Design review of the part built by this model. Coordinates are the model's own, in mm. Face numbers are marked on the shaded views. A direction names the side the tool comes from. Give positions to 0.01 mm unless a question says otherwise; leave off trailing zeros. Loops run counter-clockwise (first coordinate to the right, second up) from the corner with the lowest first, then second, coordinate; pieces in that order, holes last.
from build123d import *

# Parameters (mm, degrees)
F0_W                 = 400
F0_H                 = 200
F1_DEPTH             = 3.6
F3_W                 = 400
F3_H                 = 200
F3_W_2               = 380
F3_H_2               = 180
F4_DEPTH             = 56.4
F7_D                 = 4.2
F7_DEPTH             = 12
F7_CBORE_D           = 8
F7_CBORE_DEPTH       = 4
F7_TIP               = 1.2618073
F7_ON_F5_D           = 4.2
F7_ON_F5_DEPTH       = 12
F7_ON_F5_CBORE_D     = 8
F7_ON_F5_CBORE_DEPTH = 4
F7_ON_F5_TIP         = 1.2618073


with BuildPart() as f1:
    # F0 (on Top) → F1 (new body)
    with BuildSketch(Plane.XY):
        Rectangle(F0_W, F0_H)
    extrude(amount=-F1_DEPTH)

    # F3 (on offset) → F4 (join, through all)
    with BuildSketch(Plane.XY.offset(-60)):
        Rectangle(F3_W, F3_H)
        Rectangle(F3_W_2, F3_H_2, mode=Mode.SUBTRACT)
    extrude(amount=F4_DEPTH)

    # F7
    with Locations(Plane(origin=(-200, 0, 0), x_dir=(0, -1, 0), z_dir=(-1, 0, 0))):
        with Locations((-75, -30), (75, -30)):
            CounterBoreHole(F7_D / 2, F7_CBORE_D / 2, F7_CBORE_DEPTH, depth=F7_DEPTH)
            with Locations((0, 0, -(F7_DEPTH + F7_TIP / 2))):  # 118° drill point
                Cone(0, F7_D / 2, F7_TIP, mode=Mode.SUBTRACT)

    # F7 on F5
    with Locations(Plane.YZ.offset(200)):
        with Locations((75, -30), (-75, -30)):
            CounterBoreHole(F7_ON_F5_D / 2, F7_ON_F5_CBORE_D / 2, F7_ON_F5_CBORE_DEPTH, depth=F7_ON_F5_DEPTH)
            with Locations((0, 0, -(F7_ON_F5_DEPTH + F7_ON_F5_TIP / 2))):  # 118° drill point
                Cone(0, F7_ON_F5_D / 2, F7_ON_F5_TIP, mode=Mode.SUBTRACT)


solid = f1.part
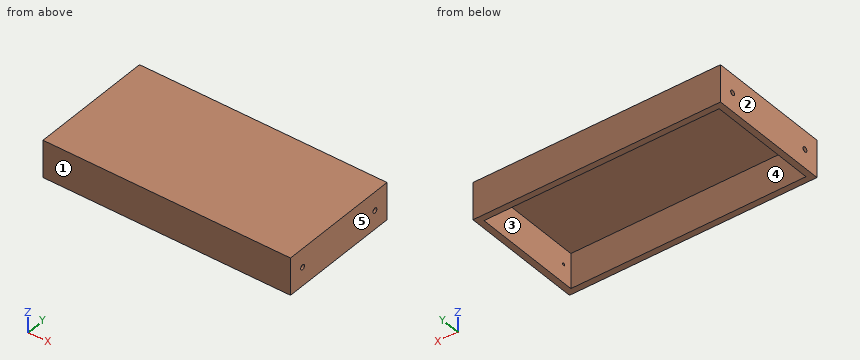
Q1. Take a section at A-A (y = -60.5). Give the boundary of the cut face in (x, z).
Results:
outline: (-200, -60) - (-190, -60) - (-190, -3.6) - (190, -3.6) - (190, -60) - (200, -60) - (200, 0) - (-200, 0) - close
Q2. Insertion check: pin 1 (4 mm diameter, centred on y = 75, z = -30, fed in from -X); pin 2 (2.5 mm diameter, centred on y = 74.5, z = -31, fed in from -X); pin 3 (6.5 mm diameter, centred on y = -75, z = -30, fed in from +X); pin 4 (8 mm diameter, centred on x = 145.5, y = 43, fed in from -Z). Each pin has a flat end and moves straight along its axis. Give the tip position at first contact, or say it passes through.
Results:
pin 1: passes through
pin 2: stops at x = -196
pin 3: stops at x = 196
pin 4: stops at z = -3.6
Q3. Wall thickness on line 1 (X direction, y = 14, z = -40); line 2 (Z direction, x = 192, y = 75); line 3 (Y direction, x = 65.5, z = -7.5): over which ranges is each line inside the solid? List them lowest first.
Results:
line 1: x = -200 to -190, 190 to 200
line 2: z = -60 to -32.1, -27.9 to 0
line 3: y = -100 to -90, 90 to 100
Q4. Draft analysis for pull direction Y (two halves, no side actions). For the marked faces 1, 2 and 3, state which applies: pulls with the +Y half, pulls with the -Y half, needs draft (parallel to the pull), parting line crosses it, or undercut.
Results:
face 1: pulls with the -Y half
face 2: needs draft
face 3: undercut
Q5. Tool access review of the marked faces 4 and 5: name each direction out of +Z, -Z, +X, -X, +Y, -Y from which nothing blocks a thin tool from reaching the whole face with its end or side.
Results:
face 4: -Z
face 5: +Z, -Z, +X, +Y, -Y
Q6. Take a section at C-C (x = -34). Give the boundary of the cut face in (y, z).
Results:
outline: (-100, -60) - (-90, -60) - (-90, -3.6) - (90, -3.6) - (90, -60) - (100, -60) - (100, 0) - (-100, 0) - close
Q7. Take a section at B-B (z = -18.5). Give the boundary of the cut face in (x, y).
Results:
outline: (-200, -100) - (200, -100) - (200, 100) - (-200, 100) - close; hole (-190, -90) - (190, -90) - (190, 90) - (-190, 90) - close
